from build123d import *

# Parameters (mm, degrees)
SKETCH1_W              = 40
SKETCH1_H              = 33.5
BOSS_EXTRUDE1_DEPTH    = 7
M3_CLEARANCE_HOLE1_D   = 3.4
SKETCH4_W              = 31.219256934
SKETCH4_H              = 27.926271275
CUT_EXTRUDE1_DEPTH     = 5
SKETCH5_W              = 8.780743066
SKETCH5_H              = 22.309556891
CUT_EXTRUDE2_DEPTH     = 5
M2_5_CLEARANCE_HOLE2_D = 2.9
SKETCH12_W             = 26.872555909
SKETCH12_H             = 5.573728725
CUT_EXTRUDE4_DEPTH     = 8
SKETCH13_W             = 8.780743066
SKETCH13_H             = 5.573728725
BOSS_EXTRUDE2_DEPTH    = 7
SKETCH14_W             = 13.127444091
SKETCH14_H             = 5.616714384
BOSS_EXTRUDE3_DEPTH    = 5
M3_CLEARANCE_HOLE2_D   = 3.4
SKETCH17_W             = 4.5
SKETCH17_H             = 33.5
CUT_EXTRUDE5_DEPTH     = 8


with BuildPart() as part:
    # Sketch1 → Boss-Extrude1 (new body)
    with BuildSketch(Plane(origin=(0, 0, 0), x_dir=(1, 0, 0), z_dir=(0, 1, 0))):
        Rectangle(SKETCH1_W, SKETCH1_H)
    extrude(amount=BOSS_EXTRUDE1_DEPTH)

    # M3 Clearance Hole1 (through all)
    with Locations(Plane(origin=(-10.5, 7, 13.75), x_dir=(0, 0, 1), z_dir=(0, 1, 0))):
        with Locations((0, 0), (-27.5, 27.5)):
            Hole(M3_CLEARANCE_HOLE1_D / 2)

    # Sketch4 → Cut-Extrude1 (cut)
    with BuildSketch(Plane(origin=(0, 7, 0), x_dir=(1, 0, 0), z_dir=(0, 1, 0))):
        with Locations((-4.390371533, 2.786864362)):
            Rectangle(SKETCH4_W, SKETCH4_H)
    extrude(amount=-CUT_EXTRUDE1_DEPTH, mode=Mode.SUBTRACT)

    # Sketch5 → Cut-Extrude2 (cut)
    with BuildSketch(Plane(origin=(0, 7, 0), x_dir=(1, 0, 0), z_dir=(0, 1, 0))):
        with Locations((15.609628467, -0.02149283)):
            Rectangle(SKETCH5_W, SKETCH5_H)
    extrude(amount=-CUT_EXTRUDE2_DEPTH, mode=Mode.SUBTRACT)

    # M2.5 Clearance Hole2 (through all)
    with Locations(Plane(origin=(-12, 2, 0), x_dir=(0, 0, 1), z_dir=(0, 1, 0))):
        with Locations((0, 0), (0, 25), (-9.75, 15.25)):
            Hole(M2_5_CLEARANCE_HOLE2_D / 2)

    # Sketch12 → Cut-Extrude4 (cut, through all)
    with BuildSketch(Plane(origin=(0, 7, 0), x_dir=(1, 0, 0), z_dir=(0, 1, 0))):
        with Locations((6.563722045, -13.963135638)):
            Rectangle(SKETCH12_W, SKETCH12_H)
    extrude(amount=-CUT_EXTRUDE4_DEPTH, mode=Mode.SUBTRACT)

    # Sketch13 → Boss-Extrude2 (add)
    with BuildSketch(Plane.XZ):
        with Locations((15.609628467, 13.963135638)):
            Rectangle(SKETCH13_W, SKETCH13_H)
    extrude(amount=-BOSS_EXTRUDE2_DEPTH)

    # Sketch14 → Boss-Extrude3 (add)
    with BuildSketch(Plane(origin=(0, 2, 0), x_dir=(1, 0, 0), z_dir=(0, 1, 0))):
        with Locations((-13.436277954, 13.941642808)):
            Rectangle(SKETCH14_W, SKETCH14_H)
    extrude(amount=BOSS_EXTRUDE3_DEPTH)

    # M3 Clearance Hole2 (through all)
    with Locations(Plane(origin=(0, 7, 0), x_dir=(1, 0, 0), z_dir=(0, 1, 0))):
        with Locations((-10.5, 13.75), (17, -13.75)):
            Hole(M3_CLEARANCE_HOLE2_D / 2)

    # Sketch17 → Cut-Extrude5 (cut, through all)
    with BuildSketch(Plane(origin=(0, 7, 0), x_dir=(1, 0, 0), z_dir=(0, 1, 0))):
        with Locations((-17.75, 0)):
            Rectangle(SKETCH17_W, SKETCH17_H)
    extrude(amount=-CUT_EXTRUDE5_DEPTH, mode=Mode.SUBTRACT)


solid = part.part
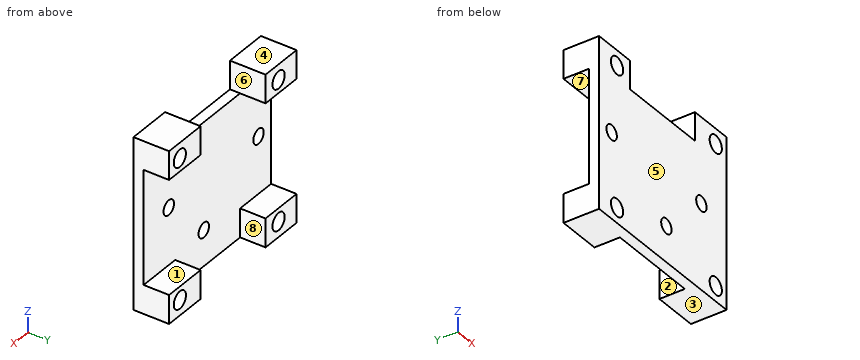
Read the model definition and answer for the solid it produces. Units are mm, in the model's axes. Face numbers are marked on the shaded views. A direction names the side the tool comes from. Round coordinates to 2 decimals unless told otherwise and drop trailing zeros. Order: outer loops, then holes, each group sorted by start corner. A loop starts at its lowest first (then second) coordinate and runs counter-clockwise, first axis right, second up.
1) The mould has two halves that part along Z. Classify the marked faces 1, 2, 3 and 4: released by +Z, released by -Z, zero draft, split by the parting line, or undercut.
2) The part is cut by section B-B on z = -13.75. Write down the section's boundary in (x, y), plus the area to 3 significant figures.
3) Flat-ended cylindrical pins translate along their axes: pin 1 (0.6 mm diameter, centred on x = 6, y = 1.5, fed in from +Z); pin 2 (4 mm diameter, centred on x = 10.5, z = 4.5, fed in from +Y); pin 3 (2.5 mm diameter, centred on x = 13, z = 0, fed in from +Y). Find the tip coordinate at first contact, or state that the pin passes through.
4) The part is cut by section D-D on z = -9.75. Write down the section's boundary in (x, y).
5) The part is cut by section A-A on y = 6. Write down the section's boundary in (x, z), plus the area to 3 significant figures.
6) The part is cut by section C-C on x = 17. Write down the section's boundary in (y, z), plus the area to 3 significant figures.
7) Straight lines are drawn through the part: L1, parallel to X at y = 2.75, z = -13.75; L2, parallel to X at y = 0.6, z = 0; L3, parallel to X at y = 1.75, z = 13. For each, find the intervals that lie inside material, in ascending order.
8) For the marked faces 5, 6, 7 and 8, determine the directions among +Z, -Z, +X, -X, +Y, -Y from which every point of the face is accessible in a straight line to the end or side of a thin tool.
Resolved:
1. face 1: undercut
1. face 2: zero draft
1. face 3: released by -Z
1. face 4: released by +Z
2. outline: (-15.5, 0) - (-12.2, 0) - (-12.2, 7) - (-15.5, 7) - close; (-8.8, 0) - (15.3, 0) - (15.3, 7) - (11.22, 7) - (11.22, 2) - (-6.87, 2) - (-6.87, 7) - (-8.8, 7) - close; (18.7, 0) - (20, 0) - (20, 7) - (18.7, 7) - close
2. area: 110 mm2
3. pin 1: stops at z = 11.18
3. pin 2: stops at y = 2
3. pin 3: passes through
4. outline: (-15.5, 0) - (1.8, 0) - (1.8, 2) - (-15.5, 2) - close; (4.7, 0) - (20, 0) - (20, 2) - (4.7, 2) - close
5. outline: (-15.5, -16.75) - (-6.87, -16.75) - (-6.87, -11.13) - (-15.5, -11.13) - close; (-15.5, 11.18) - (-6.87, 11.18) - (-6.87, 16.75) - (-15.5, 16.75) - close; (11.22, -16.75) - (20, -16.75) - (20, -11.13) - (11.22, -11.13) - close; (11.22, 11.18) - (20, 11.18) - (20, 16.75) - (11.22, 16.75) - close; hole circle Ø3.4 at (-10.5, -13.75); hole circle Ø3.4 at (-10.5, 13.75); hole circle Ø3.4 at (17, -13.75); hole circle Ø3.4 at (17, 13.75)
5. area: 158 mm2
6. outline: (0, -16.75) - (7, -16.75) - (7, -15.45) - (0, -15.45) - close; (0, -12.05) - (7, -12.05) - (7, -11.13) - (2, -11.13) - (2, 11.18) - (7, 11.18) - (7, 12.05) - (0, 12.05) - close; (0, 15.45) - (7, 15.45) - (7, 16.75) - (0, 16.75) - close
6. area: 75.4 mm2
7. L1: x = -15.5 to -12.2, -8.8 to -6.87, 11.22 to 15.3, 18.7 to 20
7. L2: x = -15.5 to -13.45, -10.55 to 11.55, 14.45 to 20
7. L3: x = -15.5 to -12.03, -8.97 to -6.87, 11.22 to 15.47, 18.53 to 20
8. face 5: +Z, -Z, +X, -X, -Y
8. face 6: +Z, +Y, -Y
8. face 7: +X, -X, +Y
8. face 8: +Z, -Z, +Y
